from build123d import *

# Parameters (mm, degrees)
SKETCH1_W           = 50
SKETCH1_H           = 80
BOSS_EXTRUDE1_DEPTH = 0.5
SKETCH4_R           = 26.335590494
BOSS_EXTRUDE2_DEPTH = 5
SKETCH5_R           = 15
BOSS_EXTRUDE3_DEPTH = 22.5
SKETCH7_R           = 10
CUT_EXTRUDE2_DEPTH  = 75.3623798


with BuildPart() as part:
    # Sketch1 → Boss-Extrude1 (new body)
    with BuildSketch(Plane(origin=(0, 0, 0), x_dir=(1, 0, 0), z_dir=(0, 1, 0))):
        Rectangle(SKETCH1_W, SKETCH1_H)
    extrude(amount=BOSS_EXTRUDE1_DEPTH)

    # Sketch4 → Boss-Extrude2 (add)
    with BuildSketch(Plane.XZ):
        with Locations(Location((0, 0, 0), (0, 0, 161.674514968))):
            Circle(SKETCH4_R)
    extrude(amount=BOSS_EXTRUDE2_DEPTH)

    # Sketch5 → Boss-Extrude3 (add, symmetric)
    with BuildSketch(Plane.XY):
        with Locations((0, 15.495084895)):
            Circle(SKETCH5_R)
    extrude(amount=BOSS_EXTRUDE3_DEPTH, both=True)

    # Sketch7 → Cut-Extrude2 (cut, through all)
    with BuildSketch(Plane.XY.offset(22.5)):
        with Locations((0, 15.498342616)):
            Circle(SKETCH7_R)
    extrude(amount=-CUT_EXTRUDE2_DEPTH, mode=Mode.SUBTRACT)


solid = part.part
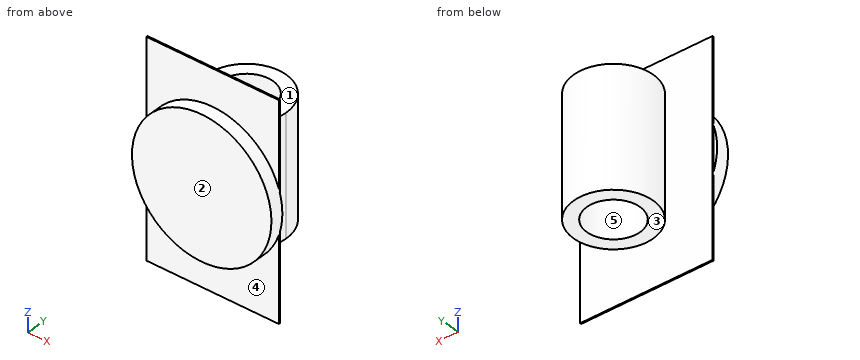
Part model, mm, in its own coordinate system. Face numbers are marked on the shaded views. A direction names the side the tool comes from. Give positions to 0.01 mm unless a question says otherwise; leave off trailing zeros. Loops run counter-clockwise (first coordinate to the right, second up) from the corner with the lowest first, then second, coordinate; pieces in that order, holes last.
(1) 3-axis set-ups, long thin cutter, end or side, ignore diameter. For the marked faces 1 and 2: which of +Z, -Z, +X, -X, +Y, -Y reach the whole face in a straight line?
Return value:
face 1: +Z, +X, -X, +Y
face 2: +Z, -Z, +X, -X, -Y
(2) Drill centre lines: line 1 along Y through (x, z) = (-2.5, 18); line 2 along Y through (x, z) = (8.5, -7.5); line 3 along Y through (x, z) = (13, 32). Where is each one in solid material? Low to high.
Return value:
line 1: y = -5 to 0.5, 0.7 to 5.82, 25.18 to 30.29
line 2: y = -5 to 0.5, 3.14 to 10.23, 20.77 to 27.85
line 3: y = 0 to 0.5
(3) Band-saw the part on A-A (y = 10). Write the cut outline in (x, z), and give its area (3 significant figures).
Return value:
outline: (-13.96, -22.5) - (-8.35, -22.5) - (-8.35, 22.5) - (-13.96, 22.5) - close; (8.35, -22.5) - (13.96, -22.5) - (13.96, 22.5) - (8.35, 22.5) - close
area: 504 mm2
(4) Pull direction Y, two halves, no side cores. Call the marked faces 3, 4 and 5: pulls with the +Y half, pulls with the -Y half, needs draft (parallel to the pull), parting line crosses it, or undercut.
Return value:
face 3: needs draft
face 4: pulls with the -Y half
face 5: undercut
(5) Band-saw the part on D-D (z = 21). Write the cut outline in (x, y).
Return value:
outline: (-25, 0) - (-15.89, 0) - (-15.89, -5) - (15.89, -5) - (15.89, 0) - (25, 0) - (25, 0.5) - (0.38, 0.5) arc R15 ccw (long way) to (-0.38, 0.5) - (-25, 0.5) - close; hole circle Ø20 at (0, 15.5)
(6) Pin check, flat tips, straight feed: pin 1 (5 mm diameter, centred on y = -0.5, z = -13, fed in from -X); pin 2 (1.1 mm diameter, centred on x = 25.5, z = -4, fed in from +Y); pin 3 (1 mm diameter, centred on x = 7, z = 6, fed in from +Y); pin 4 (16 mm diameter, centred on x = 0, y = 15.5, fed in from -Z). Stop position of each tip, or through.
Return value:
pin 1: stops at x = -25
pin 2: stops at y = 0.5
pin 3: stops at y = 29.01
pin 4: passes through
(7) Band-saw the part on C-C (y = 19). Write the cut outline in (x, z).
Return value:
outline: (-14.58, -22.5) - (-9.37, -22.5) - (-9.37, 22.5) - (-14.58, 22.5) - close; (9.37, -22.5) - (14.58, -22.5) - (14.58, 22.5) - (9.37, 22.5) - close
(8) Band-saw the part on B-B (z = -18). Write the cut outline in (x, y).
Return value:
outline: (-25, 0) - (-19.22, 0) - (-19.22, -5) - (19.22, -5) - (19.22, 0) - (25, 0) - (25, 0.5) - (0.38, 0.5) arc R15 ccw (long way) to (-0.38, 0.5) - (-25, 0.5) - close; hole circle Ø20 at (0, 15.5)
